from build123d import *

# Parameters (mm, degrees)
SKETCH1_W           = 30
SKETCH1_H           = 30
BOSS_EXTRUDE1_DEPTH = 10
SKETCH2_W           = 30
SKETCH2_H           = 2.5
BOSS_EXTRUDE2_DEPTH = 30
SKETCH3_W           = 30
SKETCH3_H           = 7.112
BOSS_EXTRUDE3_DEPTH = 30
CUT_EXTRUDE2_REACH  = 55.205
SKETCH4_R           = 11.1506
FILLET2_R           = 1
SKETCH5_R           = 3.875
CUT_EXTRUDE3_DEPTH  = 30
SKETCH6_R           = 3
CUT_EXTRUDE4_DEPTH  = 30
FILLET3_R           = 1
FILLET4_R           = 10
FILLET5_R           = 10
FILLET6_R           = 10
FILLET7_R           = 10


with BuildPart() as part:
    # Sketch1 → Boss-Extrude1 (new body)
    with BuildSketch(Plane(origin=(0, 0, 0), x_dir=(1, 0, 0), z_dir=(0, 1, 0))):
        with Locations((3.18772861, 17.116506927)):
            Rectangle(SKETCH1_W, SKETCH1_H)
    extrude(amount=BOSS_EXTRUDE1_DEPTH)

    # Sketch2 → Boss-Extrude2 (add)
    with BuildSketch(Plane(origin=(0, 10, 0), x_dir=(1, 0, 0), z_dir=(0, 1, 0))):
        with Locations((3.18772861, 30.866506927)):
            Rectangle(SKETCH2_W, SKETCH2_H)
    extrude(amount=BOSS_EXTRUDE2_DEPTH)

    # Sketch3 → Boss-Extrude3 (add)
    with BuildSketch(Plane(origin=(0, 10, 0), x_dir=(1, 0, 0), z_dir=(0, 1, 0))):
        with Locations((3.18772861, 5.672506927)):
            Rectangle(SKETCH3_W, SKETCH3_H)
    extrude(amount=BOSS_EXTRUDE3_DEPTH)

    # Sketch4 → Cut-Extrude2 (cut, up to next)
    with BuildSketch(Plane.XY.offset(-2.116506927), mode=Mode.PRIVATE) as cut_extrude2_sk1:
        with Locations((3.18772861, 25)):
            Circle(SKETCH4_R)
    cut_extrude2_tool1 = extrude(cut_extrude2_sk1.sketch, amount=-CUT_EXTRUDE2_REACH, mode=Mode.PRIVATE) & part.part
    add(cut_extrude2_tool1.solids().sort_by_distance((3.187729, 25, -2.116507))[0], mode=Mode.SUBTRACT)

    # Fillet2
    fillet2_edges = [part.edges().sort_by_distance(p)[0] for p in [
        (-7.96287139, 25, -2.116506927),
    ]]
    fillet(fillet2_edges, radius=FILLET2_R)

    # Sketch5 → Cut-Extrude3 (cut)
    with BuildSketch(Plane(origin=(0, 0, -32.116506927), x_dir=(-1, 0, 0), z_dir=(0, 0, -1))):
        with Locations((-3.18772861, 25)):
            Circle(SKETCH5_R)
    extrude(amount=-CUT_EXTRUDE3_DEPTH, mode=Mode.SUBTRACT)

    # Sketch6 → Cut-Extrude4 (cut)
    with BuildSketch(Plane(origin=(0, 0, 0), x_dir=(-1, 0, 0), z_dir=(0, -1, 0))):
        with Locations(Location((-3.18772861, 17.116506927, 0), (0, 0, 90))):
            Circle(SKETCH6_R)
    extrude(amount=-CUT_EXTRUDE4_DEPTH, mode=Mode.SUBTRACT)

    # Fillet3
    fillet3_edges = [part.edges().sort_by_distance(p)[0] for p in [
        (3.18772861, 0, -14.116506927),
    ]]
    fillet(fillet3_edges, radius=FILLET3_R)

    # Fillet4
    fillet4_edges = [part.edges().sort_by_distance(p)[0] for p in [
        (-11.81227139, 40, -30.866506927),
        (18.18772861, 40, -30.866506927),
    ]]
    fillet(fillet4_edges, radius=FILLET4_R)

    # Fillet5
    fillet5_edges = [part.edges().sort_by_distance(p)[0] for p in [
        (18.18772861, 10, -19.422506927),
    ]]
    fillet(fillet5_edges, radius=FILLET5_R - 0.0001)  # a hair under: the kernel refuses the full size

    # Fillet6
    fillet6_edges = [part.edges().sort_by_distance(p)[0] for p in [
        (-11.81227139, 10, -19.422506927),
    ]]
    fillet(fillet6_edges, radius=FILLET6_R - 0.0001)  # a hair under: the kernel refuses the full size

    # Fillet7
    fillet7_edges = [part.edges().sort_by_distance(p)[0] for p in [
        (-11.81227139, 40, -5.672506927),
        (18.18772861, 40, -5.672506927),
    ]]
    fillet(fillet7_edges, radius=FILLET7_R)


solid = part.part
The listing builds one solid part. Answer for the finished solid, in the listing's coordinates (mm). A direction names the side the tool comes from. Coordinates: 2 decimals unless noted, no trailing zeros. Write each loop counter-clockwise with the first axis right and the second up, starting at its lowest first coordinate (ties: lowest second). Pieces come first, ordered by that corner, then holes. Notation, with made-up numbers: M 29,87.5 L 43,87.5 A21 ccw 43,115.5 Z; hole C 66.5,37 d11. An arc over 180 degrees is marked long. Put each result on its own line as item: value. Start each with the question number.
1. A cutting plane is placed at A-A on y = 25. Write down the section's boundary in (x, z).
2. A cutting plane is placed at B-B on z = -4.5. Write down the section's boundary in (x, y).
3. For a pull along Z with two mould halves and no side action, classify faces 1 (the cylindrical face through (2.04, 5.44, -19.89)), 2 (the flat face through (3, 11, -2.117)), 3 (the cylindrical face through (-8.805, 37.148, -5.722)) as pulls with the +Z half, pulls with the -Z half, needs draft (parallel to the pull), parting line crosses it, or undercut.
4. Flat-ended cylindrical pins translate along their axes: P1, Ø5, axis at x = 2, z = -16, coming from the +Y side; P2, Ø1.5, axis at x = 2.5, y = 31, coming from the +Z side. Find the tip coordinate at first contact, or state that the pin passes through.
5. A cutting plane is placed at D-D on x = 16. Write down the section's boundary in (y, z).
6. Consider line 1 (Z direction, x = -2.25, y = 13); line 2 (Y direction, x = 3.25, z = -6.5); line 3 (Z direction, x = 2.25, y = 18.5). Determine where each line is inside the solid, lowest interval first. Write a range as from..to.
7. Which of the six approach directions +Z, -Z, +X, -X, +Y, -Y give full straight-line access (tool end or side, diameter ignored) to faces 4 (the cylindrical face through (15.18, 7.15, -19.57)), 5 (the cylindrical face through (-8.961, 6.993, -19.565)), 6 (the cylindrical face through (0.77, 14.115, -6.13))?
Resolved:
1. outline: M -11.81,-32.12 L -0.69,-32.12 L -0.69,-29.62 L -11.81,-29.62 Z; M -11.81,-9.23 L -7.96,-9.23 L -7.96,-3.12 A1 ccw -8.96,-2.12 L -11.81,-2.12 Z; M 7.06,-32.12 L 18.19,-32.12 L 18.19,-29.62 L 7.06,-29.62 Z; M 14.34,-9.23 L 18.19,-9.23 L 18.19,-2.12 L 15.34,-2.12 A1 ccw 14.34,-3.12 Z
2. outline: M -11.81,0 L 18.19,0 L 18.19,30 A10 ccw 8.19,40 L -1.81,40 A10 ccw -11.81,30 Z; hole C 3.19,25 d22.3
3. face 1: undercut
3. face 2: pulls with the +Z half
3. face 3: needs draft
4. P1: stops at y = 10
4. P2: stops at z = -29.62
5. outline: M 0,-32.12 L 36.24,-32.12 L 36.24,-29.62 L 6.24,-29.62 L 6.24,-9.23 L 36.24,-9.23 L 36.24,-2.12 L 0,-2.12 Z
6. line 1: z = -32.12..-29.62, -9.23..-2.12
6. line 2: y = 0..13.85, 36.15..40
6. line 3: z = -32.12..-29.62
7. face 4: +X, +Y
7. face 5: -X, +Y
7. face 6: +Z
